from build123d import *

# Parameters (mm, degrees)
SKETCH2_R           = 65
BOSS_EXTRUDE1_DEPTH = 250


with BuildPart() as part:
    # Sketch2 → Boss-Extrude1 (new body)
    with BuildSketch(Plane(origin=(0, 0, 0), x_dir=(1, 0, 0), z_dir=(0, 1, 0))):
        with BuildLine():
            Line((-11.012600748, 69.128305525), (-11.799215087, 74.066041634))
            ThreePointArc((-11.799215087, 74.066041634), (-15.659361787, 73.347013494), (-19.476587264, 72.426946288))
            Line((-19.476587264, 72.426946288), (-18.178148113, 67.598483202))
            ThreePointArc((-18.178148113, 67.598483202), (-21.691066852, 66.554471066), (-25.144531884, 65.32803775))
            Line((-25.144531884, 65.32803775), (-26.940569876, 69.994326161))
            ThreePointArc((-26.940569876, 69.994326161), (-30.566868752, 68.488440884), (-34.109385966, 66.79483355))
            Line((-34.109385966, 66.79483355), (-31.835426902, 62.341844647))
            ThreePointArc((-31.835426902, 62.341844647), (-35.054517609, 60.590269806), (-38.177526321, 58.672621247))
            Line((-38.177526321, 58.672621247), (-40.904492486, 62.863522765))
            ThreePointArc((-40.904492486, 62.863522765), (-44.138456878, 60.636594763), (-47.251440827, 58.243466069))
            Line((-47.251440827, 58.243466069), (-44.101344772, 54.360568332))
            ThreePointArc((-44.101344772, 54.360568332), (-46.885917737, 51.977983012), (-49.541979661, 49.452929653))
            Line((-49.541979661, 49.452929653), (-53.080692494, 52.985281771))
            ThreePointArc((-53.080692494, 52.985281771), (-55.780982638, 50.134638485), (-58.328380986, 47.146579638))
            Line((-58.328380986, 47.146579638), (-54.439822253, 44.003474329))
            ThreePointArc((-54.439822253, 44.003474329), (-56.668178276, 41.094008942), (-58.741210761, 38.071907732))
            Line((-58.741210761, 38.071907732), (-62.937011529, 40.791329713))
            ThreePointArc((-62.937011529, 40.791329713), (-64.985611789, 37.441557932), (-66.856091005, 33.989161443))
            Line((-66.856091005, 33.989161443), (-62.399018271, 31.723217347))
            ThreePointArc((-62.399018271, 31.723217347), (-63.9737675, 28.41402949), (-65.373169079, 25.026960753))
            Line((-65.373169079, 25.026960753), (-70.042681156, 26.814600807))
            ThreePointArc((-70.042681156, 26.814600807), (-71.350057871, 23.112101633), (-72.461869036, 19.346253794))
            Line((-72.461869036, 19.346253794), (-67.631077767, 18.056503541))
            ThreePointArc((-67.631077767, 18.056503541), (-68.483396104, 14.492220604), (-69.148006213, 10.888215497))
            Line((-69.148006213, 10.888215497), (-74.087149514, 11.665945176))
            ThreePointArc((-74.087149514, 11.665945176), (-74.596164047, 7.772535588), (-74.900715679, 3.857822021))
            Line((-74.900715679, 3.857822021), (-69.907334634, 3.600633886))
            ThreePointArc((-69.907334634, 3.600633886), (-69.999971679, -0.062967864), (-69.900743667, -3.726397024))
            Line((-69.900743667, -3.726397024), (-74.893653929, -3.99256824))
            ThreePointArc((-74.893653929, -3.99256824), (-74.582059903, -7.906727558), (-74.066041634, -11.799215087))
            Line((-74.066041634, -11.799215087), (-69.128305525, -11.012600748))
            ThreePointArc((-69.128305525, -11.012600748), (-68.457212594, -14.615404334), (-67.598483202, -18.178148113))
            Line((-67.598483202, -18.178148113), (-72.426946288, -19.476587264))
            ThreePointArc((-72.426946288, -19.476587264), (-71.308361856, -23.24042877), (-69.994326161, -26.940569876))
            Line((-69.994326161, -26.940569876), (-65.32803775, -25.144531884))
            ThreePointArc((-65.32803775, -25.144531884), (-63.922544825, -28.529077502), (-62.341844647, -31.835426902))
            Line((-62.341844647, -31.835426902), (-66.79483355, -34.109385966))
            ThreePointArc((-66.79483355, -34.109385966), (-64.918146221, -37.558411724), (-62.863522765, -40.904492486))
            Line((-62.863522765, -40.904492486), (-58.672621247, -38.177526321))
            ThreePointArc((-58.672621247, -38.177526321), (-56.594155112, -41.195893086), (-54.360568332, -44.101344772))
            Line((-54.360568332, -44.101344772), (-58.243466069, -47.251440827))
            ThreePointArc((-58.243466069, -47.251440827), (-55.690696084, -50.234911861), (-52.985281771, -53.080692494))
            Line((-52.985281771, -53.080692494), (-49.452929653, -49.541979661))
            ThreePointArc((-49.452929653, -49.541979661), (-46.792329252, -52.062250462), (-44.003474329, -54.439822253))
            Line((-44.003474329, -54.439822253), (-47.146579638, -58.328380986))
            ThreePointArc((-47.146579638, -58.328380986), (-44.029295295, -60.715905296), (-40.791329713, -62.937011529))
            Line((-40.791329713, -62.937011529), (-38.071907732, -58.741210761))
            ThreePointArc((-38.071907732, -58.741210761), (-34.94545407, -60.65323767), (-31.723217347, -62.399018271))
            Line((-31.723217347, -62.399018271), (-33.989161443, -66.856091005))
            ThreePointArc((-33.989161443, -66.856091005), (-30.443603025, -68.543322321), (-26.814600807, -70.042681156))
            Line((-26.814600807, -70.042681156), (-25.026960753, -65.373169079))
            ThreePointArc((-25.026960753, -65.373169079), (-21.571294857, -66.593387346), (-18.056503541, -67.631077767))
            Line((-18.056503541, -67.631077767), (-19.346253794, -72.461869036))
            ThreePointArc((-19.346253794, -72.461869036), (-15.527379218, -73.375067255), (-11.665945176, -74.087149514))
            Line((-11.665945176, -74.087149514), (-10.888215497, -69.148006213))
            ThreePointArc((-10.888215497, -69.148006213), (-7.254366549, -69.623086444), (-3.600633886, -69.907334634))
            Line((-3.600633886, -69.907334634), (-3.857822021, -74.900715679))
            ThreePointArc((-3.857822021, -74.900715679), (0.067465569, -74.999969656), (3.99256824, -74.893653929))
            Line((3.99256824, -74.893653929), (3.726397024, -69.900743667))
            ThreePointArc((3.726397024, -69.900743667), (7.379612388, -69.609922576), (11.012600748, -69.128305525))
            Line((11.012600748, -69.128305525), (11.799215087, -74.066041634))
            ThreePointArc((11.799215087, -74.066041634), (15.659361787, -73.347013494), (19.476587264, -72.426946288))
            Line((19.476587264, -72.426946288), (18.178148113, -67.598483202))
            ThreePointArc((18.178148113, -67.598483202), (21.691066852, -66.554471066), (25.144531884, -65.32803775))
            Line((25.144531884, -65.32803775), (26.940569876, -69.994326161))
            ThreePointArc((26.940569876, -69.994326161), (30.566868752, -68.488440884), (34.109385966, -66.79483355))
            Line((34.109385966, -66.79483355), (31.835426902, -62.341844647))
            ThreePointArc((31.835426902, -62.341844647), (35.054517609, -60.590269806), (38.177526321, -58.672621247))
            Line((38.177526321, -58.672621247), (40.904492486, -62.863522765))
            ThreePointArc((40.904492486, -62.863522765), (44.138456878, -60.636594763), (47.251440827, -58.243466069))
            Line((47.251440827, -58.243466069), (44.101344772, -54.360568332))
            ThreePointArc((44.101344772, -54.360568332), (46.885917737, -51.977983012), (49.541979661, -49.452929653))
            Line((49.541979661, -49.452929653), (53.080692494, -52.985281771))
            ThreePointArc((53.080692494, -52.985281771), (55.780982638, -50.134638485), (58.328380986, -47.146579638))
            Line((58.328380986, -47.146579638), (54.439822253, -44.003474329))
            ThreePointArc((54.439822253, -44.003474329), (56.668178276, -41.094008942), (58.741210761, -38.071907732))
            Line((58.741210761, -38.071907732), (62.937011529, -40.791329713))
            ThreePointArc((62.937011529, -40.791329713), (64.985611789, -37.441557932), (66.856091005, -33.989161443))
            Line((66.856091005, -33.989161443), (62.399018271, -31.723217347))
            ThreePointArc((62.399018271, -31.723217347), (63.9737675, -28.41402949), (65.373169079, -25.026960753))
            Line((65.373169079, -25.026960753), (70.042681156, -26.814600807))
            ThreePointArc((70.042681156, -26.814600807), (71.350057871, -23.112101633), (72.461869036, -19.346253794))
            Line((72.461869036, -19.346253794), (67.631077767, -18.056503541))
            ThreePointArc((67.631077767, -18.056503541), (68.483396104, -14.492220604), (69.148006213, -10.888215497))
            Line((69.148006213, -10.888215497), (74.087149514, -11.665945176))
            ThreePointArc((74.087149514, -11.665945176), (74.596164047, -7.772535588), (74.900715679, -3.857822021))
            Line((74.900715679, -3.857822021), (69.907334634, -3.600633886))
            ThreePointArc((69.907334634, -3.600633886), (69.999971679, 0.062967864), (69.900743667, 3.726397024))
            Line((69.900743667, 3.726397024), (74.893653929, 3.99256824))
            ThreePointArc((74.893653929, 3.99256824), (74.582059903, 7.906727558), (74.066041634, 11.799215087))
            Line((74.066041634, 11.799215087), (69.128305525, 11.012600748))
            ThreePointArc((69.128305525, 11.012600748), (68.457212594, 14.615404334), (67.598483202, 18.178148113))
            Line((67.598483202, 18.178148113), (72.426946288, 19.476587264))
            ThreePointArc((72.426946288, 19.476587264), (71.308361856, 23.24042877), (69.994326161, 26.940569876))
            Line((69.994326161, 26.940569876), (65.32803775, 25.144531884))
            ThreePointArc((65.32803775, 25.144531884), (63.922544825, 28.529077502), (62.341844647, 31.835426902))
            Line((62.341844647, 31.835426902), (66.79483355, 34.109385966))
            ThreePointArc((66.79483355, 34.109385966), (64.918146221, 37.558411724), (62.863522765, 40.904492486))
            Line((62.863522765, 40.904492486), (58.672621247, 38.177526321))
            ThreePointArc((58.672621247, 38.177526321), (56.594155112, 41.195893086), (54.360568332, 44.101344772))
            Line((54.360568332, 44.101344772), (58.243466069, 47.251440827))
            ThreePointArc((58.243466069, 47.251440827), (55.690696084, 50.234911861), (52.985281771, 53.080692494))
            Line((52.985281771, 53.080692494), (49.452929653, 49.541979661))
            ThreePointArc((49.452929653, 49.541979661), (46.792329252, 52.062250462), (44.003474329, 54.439822253))
            Line((44.003474329, 54.439822253), (47.146579638, 58.328380986))
            ThreePointArc((47.146579638, 58.328380986), (44.029295295, 60.715905296), (40.791329713, 62.937011529))
            Line((40.791329713, 62.937011529), (38.071907732, 58.741210761))
            ThreePointArc((38.071907732, 58.741210761), (34.94545407, 60.65323767), (31.723217347, 62.399018271))
            Line((31.723217347, 62.399018271), (33.989161443, 66.856091005))
            ThreePointArc((33.989161443, 66.856091005), (30.443603025, 68.543322321), (26.814600807, 70.042681156))
            Line((26.814600807, 70.042681156), (25.026960753, 65.373169079))
            ThreePointArc((25.026960753, 65.373169079), (21.571294857, 66.593387346), (18.056503541, 67.631077767))
            Line((18.056503541, 67.631077767), (19.346253794, 72.461869036))
            ThreePointArc((19.346253794, 72.461869036), (15.527379218, 73.375067255), (11.665945176, 74.087149514))
            Line((11.665945176, 74.087149514), (10.888215497, 69.148006213))
            ThreePointArc((10.888215497, 69.148006213), (7.254366549, 69.623086444), (3.600633886, 69.907334634))
            Line((3.600633886, 69.907334634), (3.857822021, 74.900715679))
            ThreePointArc((3.857822021, 74.900715679), (-0.067465569, 74.999969656), (-3.99256824, 74.893653929))
            Line((-3.99256824, 74.893653929), (-3.726397024, 69.900743667))
            ThreePointArc((-3.726397024, 69.900743667), (-7.379612388, 69.609922576), (-11.012600748, 69.128305525))
        make_face()
        Circle(SKETCH2_R, mode=Mode.SUBTRACT)
    extrude(amount=BOSS_EXTRUDE1_DEPTH)


solid = part.part
Model file for the job. Use its own axes, mm. A direction names the side the tool comes from. Give positions to 0.01 mm unless a question says otherwise; leave off trailing zeros. Loops run counter-clockwise (first coordinate to the right, second up) from the corner with the lowest first, then second, coordinate; pieces in that order, holes last.
1) Flat gauge pins, fed straight in: pin 1 Ø1 at (y, z) = (33.5, 6.5) entering from +X; pin 2 Ø2 at (y, z) = (118, -19) entering from +X; pin 3 Ø8 at (y, z) = (67, 13) entering from -X. Where does each tip first touch, or does it go through?
2) Tool access for faces 1 (the flat face through (11.4, 123.25, 71.56)), 2 (the cylindrical face through (15.606, 123.25, 73.358)), 3 (the cylindrical face through (-46.83, 123.25, 52.03)): list every direction of +Z, -Z, +X, -X, +Y, -Y with a clear straight run to the whole face (end or side of a thin tool).
3) Pull direction Z, two halves, no side cores. Call faces 4 (the cylindrical face through (70, 123, 0)), 5 (the cylindrical face through (55.74, 123.25, 50.18)), 6 (the cylindrical face through (55.73, 123.25, -50.19)): +Z half, -Z half, draft (parallel to the pull), parting line (faces both ways), or undercut.
4) Saw through at A-A (z = 0). Write the cut outline in (x, y), plus the area to 3 significant figures.
5) Saw through at B-B (x = 0). Write the cut outline in (y, z), plus the area to 3 significant figures.
6) Wall check: line 1 (Z direction, x = 0, y = 108.5); line 2 (Z direction, x = -65.5, y = 46.5); line 3 (X direction, y = 13, z = 18). Give the ranges that are in metal, low to high.
Answer block:
1. pin 1: stops at x = 74.76
1. pin 2: stops at x = 72.43
1. pin 3: stops at x = -74.46
2. face 1: +Z, +Y, -Y
2. face 2: +Z, +X, +Y, -Y
2. face 3: +Y, -Y
3. face 4: undercut
3. face 5: +Z half
3. face 6: -Z half
4. outline: (-70, 0) - (-65, 0) - (-65, 250) - (-70, 250) - close; (65, 0) - (70, 0) - (70, 250) - (65, 250) - close
4. area: 2,500 mm2
5. outline: (0, -75) - (250, -75) - (250, -65) - (0, -65) - close; (0, 65) - (250, 65) - (250, 75) - (0, 75) - close
5. area: 5,000 mm2
6. line 1: z = -75 to -65, 65 to 75
6. line 2: z = -36.53 to -33.3, -25.08 to 25.21, 33.45 to 36.53
6. line 3: x = -67.65 to -62.46, 62.46 to 67.65
